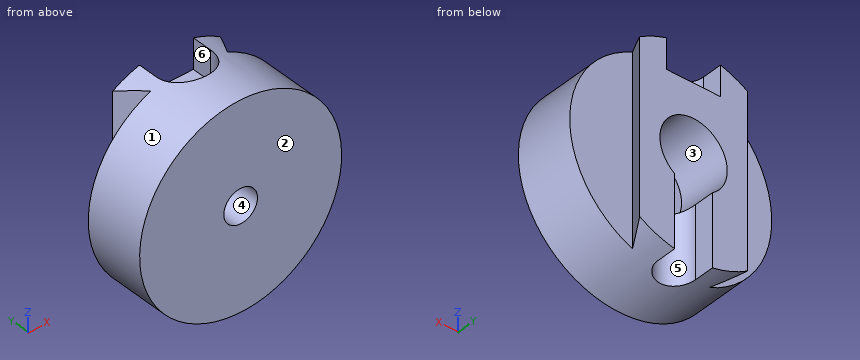
from build123d import *

# Parameters (mm, degrees)
SKETCH2_R           = 75
SKETCH2_R_2         = 12.5
BOSS_EXTRUDE1_DEPTH = 65
SKETCH3_R           = 14
CUT_EXTRUDE1_DEPTH  = 89
SKETCH4_R           = 25
CUT_EXTRUDE2_DEPTH  = 40
CUT_EXTRUDE3_DEPTH  = 97.5
SKETCH7_R           = 20
CUT_EXTRUDE4_DEPTH  = 73


with BuildPart() as part:
    # Sketch2 → Boss-Extrude1 (new body)
    with BuildSketch(Plane(origin=(0, 0, 0), x_dir=(1, 0, 0), z_dir=(0, 1, 0))):
        with Locations(Location((0, 0, 0), (0, 0, 270))):
            Circle(SKETCH2_R)
        with Locations(Location((0, 0, 0), (0, 0, 270))):
            Circle(SKETCH2_R_2, mode=Mode.SUBTRACT)
    extrude(amount=BOSS_EXTRUDE1_DEPTH)

    # Sketch3 → Cut-Extrude1 (cut)
    with BuildSketch(Plane.XY):
        with BuildLine():
            Line((-14, 77.852422798), (-14, 50))
            ThreePointArc((-14, 50), (0, 64), (14, 50))
            Line((14, 50), (14, 77.852422798))
            Line((14, 77.852422798), (-14, 77.852422798))
        make_face()
        with Locations((0, 50)):
            Circle(SKETCH3_R)
    extrude(amount=-CUT_EXTRUDE1_DEPTH, mode=Mode.SUBTRACT)

    # Sketch4 → Cut-Extrude2 (cut)
    with BuildSketch(Plane(origin=(0, 65, 0), x_dir=(1, 0, 0), z_dir=(0, 1, 0))):
        with Locations(Location((0, 0, 0), (0, 0, 270))):
            Circle(SKETCH4_R)
    extrude(amount=-CUT_EXTRUDE2_DEPTH, mode=Mode.SUBTRACT)

    # Sketch5 → Cut-Extrude3 (cut, symmetric)
    with BuildSketch(Plane.XY):
        Polygon((-75, 65), (-40, 65), (-28.452994616, 45), (-75, 45), align=None)
        Polygon((75, 65), (40, 65), (28.452994616, 45), (75, 45), align=None)
    extrude(amount=CUT_EXTRUDE3_DEPTH, both=True, mode=Mode.SUBTRACT)

    # Sketch7 → Cut-Extrude4 (cut)
    with BuildSketch(Plane.XY.offset(50)):
        with Locations((0, 50)):
            Circle(SKETCH7_R)
        with BuildLine():
            Line((-20, 82.212313003), (-20, 50))
            ThreePointArc((-20, 50), (0, 70), (20, 50))
            Line((20, 50), (20, 82.212313003))
            Line((20, 82.212313003), (-20, 82.212313003))
        make_face()
    extrude(amount=CUT_EXTRUDE4_DEPTH, mode=Mode.SUBTRACT)


solid = part.part
Input: part model. Units: mm. Frame: model coordinates. Face numbers are marked on the shaded views. A direction names the side the tool comes from. Give positions to 0.01 mm unless a question says otherwise; leave off trailing zeros. Order: outer loops, then holes, each group sorted by start corner. A loop starts at its lowest first (then second) coordinate and runs counter-clockwise, first axis right, second up. Notation, with made-up numbers: (27.25, -40) - (68.25, -40) arc R15 ccw to (68.25, -33) - close; hole circle Ø10 at (-30.5, 19). An arc over 180 degrees is marked (long way). Write each question's results on one line, items separated by ' | '.
Item 1: Section D-D (z = 52.5). Return loops of the section in (x, y).
A:
outline: (-53.56, 0) - (53.56, 0) - (53.56, 45) - (28.45, 45) - (40, 65) - (20, 65) - (20, 50) arc R20 cw to (-20, 50) - (-20, 65) - (-40, 65) - (-28.45, 45) - (-53.56, 45) - close
Item 2: Material intervals for line 1 along X through (y, z) = (16.75, 0); line 2 along X through (y, z) = (41, 0), sorted ascending.
A:
line 1: x = -75 to -12.5, 12.5 to 75 | line 2: x = -75 to -25, 25 to 75
Item 3: Section A-A (x = 0). Return loops of the section in (y, z), and give its area (3 significant figures).
A:
outline: (0, -75) - (36, -75) - (36, -25) - (25, -25) - (25, -12.5) - (0, -12.5) - close; (0, 12.5) - (25, 12.5) - (25, 25) - (65, 25) - (65, 50) - (30, 50) - (30, 75) - (0, 75) - close | area: 4,800 mm^2
Item 4: Section B-B (z = 0). Return loops of the section in (x, y).
A:
outline: (-75, 0) - (-12.5, 0) - (-12.5, 25) - (-25, 25) - (-25, 65) - (-40, 65) - (-28.45, 45) - (-75, 45) - close; (12.5, 0) - (75, 0) - (75, 45) - (28.45, 45) - (40, 65) - (25, 65) - (25, 25) - (12.5, 25) - close
Item 5: Section C-C (y = 34). Return loops of the section in (x, z), and give its area (3 significant figures).
A:
outline: (-12, 50) - (-12, 74.03) arc R75 ccw (long way) to (12, 74.03) - (12, 50) - close; hole circle Ø50 at (0, 0) | area: 15,100 mm^2
Item 6: Access query for the marked faces 4, 5 and 6. Directions: +Z, -Z, +X, -X, +Y, -Y. A direction counts if a zero-diameter tool reaches every point of the face in a straight line with its end or side. Return the directions, or none.
A:
face 4: +Y, -Y | face 5: -Z, +Y | face 6: +Z, +Y
Item 7: Draft query along X for the marked faces 1, 2 and 3. Return one class per face: released by +X, released by -X, zero draft, split by the parting line, or undercut.
A:
face 1: split by the parting line | face 2: zero draft | face 3: undercut
Item 8: Contact query for flat-ended pins moving along their axis: pin 1 Ø2 at (x, z) = (27.5, 15) entering from -Y; pin 2 Ø4.5 at (y, z) = (59.5, -60) entering from +X; pin 3 Ø5 at (y, z) = (10.5, 31.5) entering from +X; pin 4 Ø10 at (y, z) = (13, 55) entering from -X. Output: stop coordinate, or through.
A:
pin 1: stops at y = 0 | pin 2: stops at x = 38.12 | pin 3: stops at x = 69.17 | pin 4: stops at x = -55.9
